Work out the finished part from the listing and answer in its coordinate system (mm). A direction names the side the tool comes from. Give positions to 0.01 mm unless a question says otherwise; leave off trailing zeros. Write each loop counter-clockwise with the first axis right and the second up, starting at its lowest first coordinate (ties: lowest second). Pieces come first, ordered by that corner, then holes. Notation, with made-up numbers: (-30, -39) - (11, -39) arc R28 cw to (11, -18) - close; hole circle Ø2 at (86, 27.25). An arc over 180 degrees is marked (long way). Write item = value, one per line.
from build123d import *

# Parameters (mm, degrees)
SKETCH1_R               = 2.15
BOSS_EXTRUDE1_DEPTH     = 31.3
CUT_EXTRUDE1_REACH      = 48.052
SKETCH2_W               = 57.6
SKETCH2_H               = 12
CUT_EXTRUDE3_DEPTH      = 70.673542324
CUT_EXTRUDE4_DEPTH      = 41.650746822
CUT_EXTRUDE4_DEPTH_BACK = 41.650746822
SKETCH9_W               = 62.6
SKETCH9_H               = 53.637858301
SKETCH9_W_2             = 61.6
SKETCH9_H_2             = 51.637858301
SKETCH10_R              = 1.25
CUT_EXTRUDE5_DEPTH      = 12
CUT_EXTRUDE6_START      = -12
SKETCH11_R              = 1.25
CUT_EXTRUDE6_DEPTH      = 12
CORTE_EXTRUS_O1_DEPTH   = 69.776467632
FILETE1_R               = 1
FILETE2_R               = 0.35


with BuildPart() as part:
    # Sketch1 → Boss-Extrude1 (new, symmetric)
    with BuildSketch(Plane(origin=(0, 0, 0), x_dir=(0, 0, -1), z_dir=(1, 0, 0))):
        with BuildLine():
            Line((-4.25, 0), (-4.25, -4))
            ThreePointArc((-4.25, -4), (-4.121120876, -4.608298893), (-3.756629943, -5.112068414))
            Line((-3.756629943, -5.112068414), (-1.943370057, -6.753407807))
            ThreePointArc((-1.943370057, -6.753407807), (-1.578879124, -7.257177328), (-1.45, -7.865476221))
            Line((-1.45, -7.865476221), (-1.45, -21.2))
            Line((-1.45, -21.2), (22.05, -21.2))
            Line((22.05, -21.2), (12.593870957, -13.812062296))
            Line((12.593870957, -13.812062296), (3.709335443, 2.074447052))
            ThreePointArc((3.709335443, 2.074447052), (-1.071873212, 4.112613259), (-4.25, 0))
        make_face()
        Circle(SKETCH1_R, mode=Mode.SUBTRACT)
    extrude(amount=BOSS_EXTRUDE1_DEPTH, both=True)

    # Cut-Extrude1: up to this plane
    cut_extrude1_end = Plane(origin=(31.3, -13.812062296, -12.593870957), z_dir=(0, -0.4881051886126717, 0.8727848101619254))
    # Sketch2 → Cut-Extrude1 (cut, up to the surface)
    with BuildSketch(Plane.XY.offset(4.25), mode=Mode.PRIVATE) as cut_extrude1_sk1:
        with Locations((0, -1.75)):
            Rectangle(SKETCH2_W, SKETCH2_H)
    cut_extrude1_tool1 = split(extrude(cut_extrude1_sk1.sketch, amount=-CUT_EXTRUDE1_REACH, mode=Mode.PRIVATE), bisect_by=cut_extrude1_end, keep=Keep.BOTH, mode=Mode.PRIVATE)
    add(cut_extrude1_tool1.solids().sort_by_distance((0, -1.75, 4.25))[0], mode=Mode.SUBTRACT)

    # Sketch8 → Cut-Extrude3 (cut, through all)
    with BuildSketch(Plane(origin=(31.3, 0, 0), x_dir=(0, 0, -1), z_dir=(1, 0, 0))):
        with BuildLine():
            Line((-1.45, -7.865476221), (9.203660648, -7.75))
            Line((9.203660648, -7.75), (3.709335443, 2.074447052))
            ThreePointArc((3.709335443, 2.074447052), (-1.071873212, 4.112613259), (-4.25, 0))
            Line((-4.25, 0), (-4.25, -4))
            ThreePointArc((-4.25, -4), (-4.121120876, -4.608298893), (-3.756629943, -5.112068414))
            Line((-3.756629943, -5.112068414), (-1.943370057, -6.753407807))
            ThreePointArc((-1.943370057, -6.753407807), (-1.578879124, -7.257177328), (-1.45, -7.865476221))
        make_face()
    extrude(amount=-CUT_EXTRUDE3_DEPTH, mode=Mode.SUBTRACT)

    # Sketch9 → Cut-Extrude4 (cut, two sides: drawn at the far end of the back side and taken through both)
    with BuildSketch(Plane(origin=(0, -7.851819352, 0.190038007), x_dir=(1, 0, 0), z_dir=(0, 0.9999412620012955, 0.010838475319740372)).offset(-CUT_EXTRUDE4_DEPTH_BACK)):
        with Locations((0, 0.275128594)):
            Rectangle(SKETCH9_W, SKETCH9_H)
        with Locations((0, 0.275128594)):
            Rectangle(SKETCH9_W_2, SKETCH9_H_2, mode=Mode.SUBTRACT)
    extrude(amount=CUT_EXTRUDE4_DEPTH + CUT_EXTRUDE4_DEPTH_BACK, mode=Mode.SUBTRACT)

    # Sketch10 → Cut-Extrude5 (cut)
    with BuildSketch(Plane(origin=(30.8, 0, 0), x_dir=(0, 0, -1), z_dir=(1, 0, 0))):
        with Locations(Location((3.05, -11.365476221, 0), (0, 0, 90))):
            Circle(SKETCH10_R)
        with Locations(Location((7.05, -17.365476221, 0), (0, 0, 90))):
            Circle(SKETCH10_R)
    extrude(amount=-CUT_EXTRUDE5_DEPTH, mode=Mode.SUBTRACT)

    # Sketch11 → Cut-Extrude6 (cut)
    with BuildSketch(Plane.ZY.offset(30.8).offset(CUT_EXTRUDE6_START)):
        with Locations(Location((-7.05, -17.365476221, 0), (0, 0, 90))):
            Circle(SKETCH11_R)
        with Locations(Location((-3.05, -11.365476221, 0), (0, 0, 90))):
            Circle(SKETCH11_R)
    extrude(amount=CUT_EXTRUDE6_DEPTH, mode=Mode.SUBTRACT)

    # Esboço1 → Corte-extrusão1 (cut, through all)
    with BuildSketch(Plane(origin=(30.8, 0, 0), x_dir=(0, 0, -1), z_dir=(1, 0, 0))):
        with BuildLine():
            Line((-1.45, -21.2), (22.05, -21.2))
            Line((22.05, -21.2), (2.813375457, -20.2))
            ThreePointArc((2.813375457, -20.2), (0.573558931, -19.757329107), (-1.45, -18.7))
            Line((-1.45, -18.7), (-1.45, -21.2))
        make_face()
    extrude(amount=-CORTE_EXTRUS_O1_DEPTH, mode=Mode.SUBTRACT)

    # Filete1
    filete1_edges = [part.edges().sort_by_distance(p)[0] for p in [
        (0, -18.7, 1.45),
    ]]
    fillet(filete1_edges, radius=FILETE1_R)

    # Filete2
    filete2_edges = [part.edges().sort_by_distance(p)[0] for p in [
        (0, -21.2, -22.05),
    ]]
    fillet(filete2_edges, radius=FILETE2_R)


solid = part.part
1. Find section D-D, the plane y = -13.25. Give the vertices of the cut face in (x, z).
Solution:
outline = (-30.8, -12.28) - (30.8, -12.28) - (30.8, 1.45) - (-30.8, 1.45) - close
2. Find section B-B, the plane x = -11.5. Give the vertices of the cut face in (y, z), then the cut area to 3 significant figures.
Solution:
outline = (-21.14, -20.94) arc R0.35 ccw to (-20.52, -21.18) - (-13.81, -12.59) - (-7.75, -9.2) - (-7.87, 1.45) - (-18.17, 1.45) arc R1 ccw to (-19.02, 0.98) arc R8 ccw to (-20.2, -2.81) - close
area = 197 mm^2
3. For a pull along Y with two mould halves and no side action, classify faces 1 (the cylindrical face through (24.884, -18.614, -6.995)), 2 (the flat face through (30.8, -15, -7)), 3 (the flat face through (0.43, -17.21, -16.94)) as pulls with the +Y half, pulls with the -Y half, needs draft (parallel to the pull), parting line crosses it, or undercut.
Solution:
face_1 = undercut
face_2 = needs draft
face_3 = pulls with the +Y half
4. Straight lines are drawn through the part: line 1 (Y direction, x = -27.75, z = -7.05); line 2 (Y direction, x = 13, z = 0.25); line 3 (Z direction, x = 18.5, y = -8.5). For each, find the intervals that lie inside material, in ascending order.
Solution:
line_1 = -20.42 to -18.62, -16.12 to -7.77
line_2 = -19.41 to -7.85
line_3 = -9.62 to 1.45
5. Find section C-C, the plane z = -7.05. Give the vertices of the cut face in (x, y), then the cut area to 3 significant figures.
Solution:
outline = (-30.8, -20.42) - (30.8, -20.42) - (30.8, -18.62) - (18.8, -18.62) - (18.8, -16.12) - (30.8, -16.12) - (30.8, -7.77) - (-30.8, -7.77) - (-30.8, -16.12) - (-18.8, -16.12) - (-18.8, -18.62) - (-30.8, -18.62) - close
area = 719 mm^2
6. Given pin 1 (0.8 mm diameter, centred on y = -17.5, z = -7, fed in from +X); pin 2 (2 mm diameter, centred on y = -15.5, z = -18.5, fed in from +X); pin 3 (2 mm diameter, centred on x = -3, y = -13.5, fed in from -Z); pin 4 (6 mm diameter, centred on x = 15.5, y = -17, fed in from -Z), each flat-ended and moving along its own axis, determine where each tip first touches the part or whether it passes through.
Solution:
pin_1 = 18.8
pin_2 = through
pin_3 = -13.47
pin_4 = -20.51
7. Find section A-A, the plane x = 24. Give the vertices of the cut face in (y, z), then the cut area to 3 significant figures.
Solution:
outline = (-21.14, -20.94) arc R0.35 ccw to (-20.52, -21.18) - (-13.81, -12.59) - (-7.75, -9.2) - (-7.87, 1.45) - (-18.17, 1.45) arc R1 ccw to (-19.02, 0.98) arc R8 ccw to (-20.2, -2.81) - close; hole circle Ø2.5 at (-17.37, -7.05); hole circle Ø2.5 at (-11.37, -3.05)
area = 187 mm^2
8. A tool of negligible diameter and unlimited length cuts with its end or side. For faces 4 (the flat face through (-30.8, -15, -7)), 5 (the flat face through (18.8, -11, -3)), 6 (the flat face through (-18.8, -17, -7)), from which of +Z, -Z, +X, -X, +Y, -Y can it reach the whole face along a straight path? Write none if from no direction.
Solution:
face_4 = +Z, -Z, -X, +Y, -Y
face_5 = +X
face_6 = -X
